Autodesk Fusion 360 part; units mm, degrees
sketch "スケッチ1" plane through (0, 0, 0) normal (0, 0, 1) x (1, 0, 0)
  line L0 (2.1072, 3.4) -> (-2.1072, 3.4) construction
  line L1 (-2.1071, -3.4) -> (2.1071, -3.4) construction
  line L2 (17.7, 3.4) -> (-17.7, 3.4) construction
  line L3 (-17.7, 3.4) -> (-17.7, -3.4) construction
  line L4 (-17.7, -3.4) -> (17.7, -3.4) construction
  line L5 (17.7, -3.4) -> (17.7, 3.4) construction
  line L6 (17.7, 3.4) -> (-17.7, -3.4) construction
  line L7 (-17.7, 3.4) -> (17.7, -3.4) construction
  line L8 (-2.1072, 3.4) -> (-15.3703, 2.4942)
  line L9 (-2.1071, -3.4) -> (-15.3703, -2.4942)
  line L10 (2.1072, 3.4) -> (15.3703, 2.4942)
  line L11 (2.1071, -3.4) -> (15.3703, -2.4942)
  arc A0 (-15.3703, 2.4942) -> (-15.3703, -2.4942) centre (-15.2, 0) ccw
  arc A1 (15.3703, -2.4942) -> (15.3703, 2.4942) centre (15.2, 0) ccw
  arc A2 (2.1072, 3.4) -> (-2.1072, 3.4) centre (0, 0) ccw
  arc A3 (-2.1072, 3.4) -> (-2.1071, -3.4) centre (0, 0) ccw
  arc A4 (2.1071, -3.4) -> (2.1072, 3.4) centre (0, 0) ccw
  arc A5 (-2.1071, -3.4) -> (2.1071, -3.4) centre (0, 0) ccw
  line L12 (-2.1072, 3.4) -> (2.1072, 3.4)
  line L13 (-2.1071, -3.4) -> (2.1071, -3.4)
  circle A6 centre (-15.2, 0) radius 0.6
  circle A7 centre (-12.7, 0) radius 0.6
  circle A8 centre (-10.2, 0) radius 0.6
  line L14 (0, 1.75) -> (0, 22.5) construction
  circle A9 centre (10.2, 0) radius 0.6
  circle A10 centre (12.7, 0) radius 0.6
  circle A11 centre (15.2, 0) radius 0.6
  dimension "d1" = 8
  dimension "d5" = 6.8
  dimension "d6" = 35.4
  dimension "d7" = 6.8
  dimension "d8" = 2.5
  dimension "d9" = 2.5
  dimension "d10" = 1.2
  dimension "d11" = 2.5
  dimension "d14" = 2.5
  dimension "d15" = 0
extrude "押し出し1" add sketch "スケッチ1" along normal blind 5.5 contours A3 A4 L12 L13 | A2 L12 | A5 L13 makes body 1
extrude "押し出し2" add sketch "スケッチ1" along normal blind 2 contours L8 L9 A0 A3 | L10 L11 A1 A4 bodies 1
sketch "スケッチ2" plane through (0, 0, 5.5) normal (0, 0, 1) x (-1, 0, 0)
  circle A0 centre (0, 0) radius 4
  circle A1 centre (0, 0) radius 1
  circle A2 centre (0, 0) radius 2.35
  dimension "d23" = 2
  dimension "d24" = 4.7
extrude "押し出し3" cut sketch "スケッチ2" against normal through all contours A1 bodies 1
extrude "押し出し4" cut sketch "スケッチ2" against normal blind 2.6 contours A2 bodies 1
sketch "スケッチ3" plane through (0, 0, 0) normal (0, 0, 1) x (1, 0, 0)
  circle A0 centre (0, 0) radius 3.1
  dimension "d28" = 6.2
extrude "押し出し5" cut sketch "スケッチ3" along normal blind 2.1 bodies 1
copy_body "ボディ -> コンポーネント1" bodies 1 removing the originals makes body 2 in component "Component'"
component "Component'" placed x (1, 0, 0) y (0, 1, 0) z (0, 0, 1) at (0, 0, 0)
Check sheet for the modelled part. Datum: model origin and axes. Units: mm. A direction names the side the tool comes from. Round coordinates to 2 decimals unless told otherwise and drop trailing zeros. Loops run counter-clockwise (first coordinate to the right, second up) from the corner with the lowest first, then second, coordinate; pieces in that order, holes last. Notation, with made-up numbers: (26, 57) - (76, 57) arc R22 cw to (76, 95) - close; hole circle Ø10 at (9.25, 42.5). An arc over 180 degrees is marked (long way). Answer as CSV lines item,"result". Start each with the question number.
Item 1: Scan lines: line 1 (Y direction, x = 0, z = 2.75); line 2 (Z direction, x = 5.5, y = -2.75); line 3 (Y direction, x = 0, z = 4.45). Record each from-to range of solid material in increasing order. Write a range as [from, to].
Item 2: Set-up check for faces 4 (the cylindrical face through (-4, 0, 4)), 5 (the cylindrical face through (0.509, 2.294, 4.218)), 6 (the cylindrical face through (1.43, 2.75, 1.04)): record each of +Z, -Z, +X, -X, +Y, -Y from which the full face is reachable in a straight line by a thin tool's end or side.
Item 3: Section check C-C (x = 12.7). Record the boundary of the cut face in (y, z).
Item 4: Section check A-A (x = 0). Record the boundary of the cut face in (y, z).
Item 5: Depth check by flat-ended pin: P1, Ø1.6, axis at x = -10.2, y = 0, coming from the +Z side; P2, Ø3, axis at x = 0, y = 0, coming from the +Z side; P3, Ø1, axis at y = 0.5, z = 3, coming from the -X side; P4, Ø1, axis at x = 8.5, z = 3, coming from the -Y side. Enter the tip coordinate at first touch or a pass-through.
Item 6: Release check for a two-part mould opening along X. For faces 1 (the cylindrical face through (0, -4, 3)), 2 (the flat face through (-0.2, -3.5, 0)), 3 (the cylindrical face through (15.754, 0.23, 0.986)) record: +X half, -X half, draft (parallel to the pull), parting line (faces both ways), or undercut.
Item 7: Section check D-D (y = -2). Record the boundary of the cut face in (x, z), and give its area (3 significant figures).
Item 8: Section check B-B (z = 2.6). Record the boundary of the cut face in (x, y), and give its area (3 significant figures).
Report:
1,line 1,"y = [-4, -1], [1, 4]"
1,line 2,"z = [0, 2]"
1,line 3,"y = [-4, -2.35], [2.35, 4]"
2,face 4,"+Z, -X"
2,face 5,"+Z"
2,face 6,"-Z"
3,outline,"(-2.68, 0) - (-0.6, 0) - (-0.6, 2) - (-2.68, 2) - close; (0.6, 0) - (2.68, 0) - (2.68, 2) - (0.6, 2) - close"
4,outline,"(-4, 0) - (-3.1, 0) - (-3.1, 2.1) - (-1, 2.1) - (-1, 2.9) - (-2.35, 2.9) - (-2.35, 5.5) - (-4, 5.5) - close; (1, 2.1) - (3.1, 2.1) - (3.1, 0) - (4, 0) - (4, 5.5) - (2.35, 5.5) - (2.35, 2.9) - (1, 2.9) - close"
5,P1,"stops at z = 2"
5,P2,"stops at z = 2.9"
5,P3,"stops at x = -4"
5,P4,"passes through"
6,face 1,"parting line"
6,face 2,"draft"
6,face 3,"undercut"
7,outline,"(-16.7, 0) - (-2.37, 0) - (-2.37, 2.1) - (2.37, 2.1) - (2.37, 0) - (16.7, 0) - (16.7, 2) - (3.46, 2) - (3.46, 5.5) - (1.23, 5.5) - (1.23, 2.9) - (-1.23, 2.9) - (-1.23, 5.5) - (-3.46, 5.5) - (-3.46, 2) - (-16.7, 2) - close"
7,area,"74.7 mm2"
8,outline,"(-2.11, -3.4) arc R4 ccw to (2.11, -3.4) arc R4 ccw to (2.11, 3.4) arc R4 ccw to (-2.11, 3.4) arc R4 ccw to start; hole circle Ø2 at (0, 0)"
8,area,"47.1 mm2"
